The model under review builds one solid part; all positions refer to its coordinate system, in mm. A direction names the side the tool comes from. Coordinates: 2 decimals unless noted, no trailing zeros. Write each loop counter-clockwise with the first axis right and the second up, starting at its lowest first coordinate (ties: lowest second). Pieces come first, ordered by that corner, then holes. Notation, with made-up numbers: (42, 30.5) - (85, 30.5) arc R14 cw to (85, 53.5) - close; hole circle Ø2 at (49.25, 76.25). An arc over 180 degrees is marked (long way). Put each result on its own line as item: value. Start each with the question number.
Item 1: Consider section A-A on y = 5.75. Give the boundary of the cut face in (x, z).
Item 2: For pin 1 (8 mm diameter, centred on y = 16, z = 15, fed in from +X); pin 2 (1.5 mm diameter, centred on x = 13.5, y = 10, fed in from -Z); pin 3 (7 mm diameter, centred on x = 99, y = 9, fed in from -Z), all flat-tipped, find the tip position at first contact; note any pin that passes through.
Item 3: Consider section B-B on z = 15.5. Give the boundary of the cut face in (x, y), then the cut area to 3 significant figures.
Item 4: Consider section C-C on x = 21.5. Give the boundary of the cut face in (y, z), then the cut area to 3 significant figures.
Item 5: Machinability: for faces 4 (the face through (100.6, 10.14, 113.64)), 5 (the face through (51, 10, 105.5)), which of the approach directions +Z, -Z, +X, -X, +Y, -Y give a long, thin tool a straight path to every point of the face, cutting with its end or side? Answer none if there is none.
Item 6: Mouldability with a two-part tool opening along X and no side actions: class faces 1 (the face through (97, 10, 53)), 2 (the face through (9, 10, 32)), 3 (the face through (101.5, 10, 83)) as pulls with the +X half, pulls with the -X half, needs draft (parallel to the pull), parting line crosses it, or undercut.
Item 7: To check wall thickness, follow L1, parallel to X at y = 2.75, z = 85; L2, parallel to Z at x = 72, y = 10; L3, parallel to X at y = 16.5, z = 41.5. State the ranges of each line that lie inside material, in increasing order. Write a range as [from, to].
```python
from build123d import *

# Parameters (mm, degrees)
SKETCH_1_W      = 9
SKETCH_1_H      = 105.5
EXTRUDE_1_DEPTH = 20
FILLET_1_R      = 3
SKETCH_2_W      = 40
SKETCH_2_H      = 20
EXTRUDE_2_DEPTH = 9


with BuildPart() as part:
    # 草图1 → 凸台-拉伸1 (new body)
    with BuildSketch(Plane(origin=(0, 0, 0), x_dir=(1, 0, 0), z_dir=(0, 1, 0))):
        with Locations((4.5, -52.75)):
            Rectangle(SKETCH_1_W, SKETCH_1_H)
        Polygon((9, -105.5), (0, -105.5), (0, -114.5), (92.5, -114.5), (92.5, -105.5), align=None)
        Polygon((92.5, -53), (92.5, -105.5), (92.5, -114.5), (101.5, -114.5), (101.5, -53), align=None)
    extrude(amount=EXTRUDE_1_DEPTH)

    # 圆角1
    fillet_1_edges = [part.edges().sort_by_distance(p)[0] for p in [
        (101.5, 10, 114.5),
        (0, 10, 114.5),
    ]]
    fillet(fillet_1_edges, radius=FILLET_1_R)

    # 草图2 → 凸台-拉伸2 (add)
    with BuildSketch(Plane.ZY):
        with Locations((-20, 10)):
            Rectangle(SKETCH_2_W, SKETCH_2_H)
    extrude(amount=-EXTRUDE_2_DEPTH)


solid = part.part
```
Report:
1. outline: (0, -40) - (9, -40) - (9, 105.5) - (92.5, 105.5) - (92.5, 53) - (101.5, 53) - (101.5, 111.5) arc R3 ccw to (98.5, 114.5) - (3, 114.5) arc R3 ccw to (0, 111.5) - close
2. pin 1: x = 9
2. pin 2: z = 105.5
2. pin 3: z = 53
3. outline: (0, 0) - (9, 0) - (9, 20) - (0, 20) - close
3. area: 180 mm²
4. outline: (0, 105.5) - (20, 105.5) - (20, 114.5) - (0, 114.5) - close
4. area: 180 mm²
5. face 4: +Z, +X, +Y, -Y
5. face 5: -Z, +Y, -Y
6. face 1: needs draft
6. face 2: undercut
6. face 3: pulls with the +X half
7. L1: [0, 9], [92.5, 101.5]
7. L2: [105.5, 114.5]
7. L3: [0, 9]
